```python
from build123d import *

# Parameters (mm, degrees)
F1_DEPTH = 60
F3_DEPTH = 25
F4_R     = 10
F5_DEPTH = 50.8
F7_DEPTH = 42.5
F8_R     = 20


with BuildPart() as f1:
    # F0 (on Front) → F1 (new body)
    with BuildSketch(Plane.XZ):
        with BuildLine():
            Line((94.505748464, -21.1170856844), (94.505748464, -11.1170856844))
            Line((94.505748464, -11.1170856844), (-19.3909259748, -11.1170856844))
            ThreePointArc((-19.3909259748, -11.1170856844), (-22.0195815354, -10.3703397262), (-23.8630619298, -8.3531536619))
            Line((-23.8630619298, -8.3531536619), (-60.860814682, 65.6423518426))
            Line((-60.860814682, 65.6423518426), (-69.805086592, 61.1702158876))
            Line((-69.805086592, 61.1702158876), (-42.972270862, 7.5045844276))
            Line((-42.972270862, 7.5045844276), (-55.494251536, 1.2435940906))
            Line((-55.494251536, 1.2435940906), (-82.327067266, 54.9092255506))
            Line((-82.327067266, 54.9092255506), (-91.271339176, 50.4370895956))
            Line((-91.271339176, 50.4370895956), (-55.494251536, -21.1170856844))
            Line((-55.494251536, -21.1170856844), (94.505748464, -21.1170856844))
        make_face()
    extrude(amount=F1_DEPTH)

    # F2 (on face) → F3 (cut)
    with BuildSketch(Plane.XY.offset(-11.1170856844)):
        with BuildLine():
            Line((94.505748464, -25), (29.505748464, -25))
            ThreePointArc((29.505748464, -25), (24.505748464, -30), (29.505748464, -35))
            Line((29.505748464, -35), (94.505748464, -35))
            Line((94.505748464, -35), (94.505748464, -25))
        make_face()
    extrude(amount=-F3_DEPTH, mode=Mode.SUBTRACT)

    # F4 (on face) → F5 (cut)
    with BuildSketch(Plane(origin=(-22.4317110086, 0, -11.2158555043), x_dir=(0, 1, 0), z_dir=(0.894427191, 0, 0.4472135955))):
        with Locations((-30, 51.9005979594)):
            Circle(F4_R)
    extrude(amount=-F5_DEPTH, mode=Mode.SUBTRACT)

    # F6 (on face) → F7 (cut)
    with BuildSketch(Plane(origin=(-22.4317110086, 0, -11.2158555043), x_dir=(0, 1, 0), z_dir=(0.894427191, 0, 0.4472135955))):
        with BuildLine():
            ThreePointArc((-23.0317006599, 85.9300881282), (-8.8437530091, 78.6280740539), (0, 65.346308328))
            Line((0, 65.346308328), (0, 85.9300881282))
            Line((0, 85.9300881282), (-23.0317006599, 85.9300881282))
        make_face()
        with BuildLine():
            ThreePointArc((-60, 65.346308328), (-51.1562469909, 78.6280740539), (-36.9682993401, 85.9300881282))
            Line((-36.9682993401, 85.9300881282), (-60, 85.9300881282))
            Line((-60, 85.9300881282), (-60, 65.346308328))
        make_face()
    extrude(amount=-F7_DEPTH, mode=Mode.SUBTRACT)

    # F8
    f8_edges = [f1.edges().sort_by_distance(p)[0] for p in [
        (94.505748, 0, -16.117086),
        (94.505748, -60, -16.117086),
    ]]
    fillet(f8_edges, radius=F8_R)


solid = f1.part
```
Design review of the part built by this model. Coordinates are the model's own, in mm. A direction names the side the tool comes from. Give positions to 0.01 mm unless a question says otherwise; leave off trailing zeros. Write each loop counter-clockwise with the first axis right and the second up, starting at its lowest first coordinate (ties: lowest second). Pieces come first, ordered by that corner, then holes. Notation, with made-up numbers: (-3, 66.5) - (7, 66.5) arc R21 ccw to (7, 79.5) - close; hole circle Ø7 at (-12.5, 6.5). An arc over 180 degrees is marked (long way). Return JSON: item names as keys, results as strings. Group by question number.
(1) We need section B-B, the plane y = -27.5. Give the boundary of the cut face in (x, z).
(2) Insertion check: pin 1 (2 mm diameter, centred on x = -24, y = -26.5, fed in from +Z); pin 2 (10 mm diameter, centred on x = 38, y = -26, fed in from +Z); pin 3 (4 mm diameter, centred on x = -65.5, z = 56.5, fed in from +Y); pin 4 (4 mm diameter, centred on x = -34.5, z = -11, fed in from +Y). Each pin has a flat end and moves straight along its axis. Give the tip position at first contact, or say it passes through.
(3) We need section A-A, the plane x = 65. Give the boundary of the cut face in (y, z), then the cut area to 3 significant figures.
(4) Mouldability with a two-part tool opening along X and no side actions: class faces 1 (the cylindrical face through (-21.99, -29.58, -10.39)), 2 (the flat face through (-71.704, -29.58, 33.664)), 3 (the flat face through (-65.27, -29.902, 63.438)) as +X half, -X half, draft (parallel to the pull), parting line (faces both ways), or undercut.
(5) Machinability: for faces 4 (the flat face through (-59.56, -29.58, 40.68)), 5 (the cylindrical face through (88.8, -6.01, -16.05)), 6 (the flat face through (62, -25, -16)), which of the approach directions +Z, -Z, +X, -X, +Y, -Y give a long, thin tool a straight path to every point of the face, cutting with its end or side? Answer none if there is none.
(6) We need section D-D, the plane y = -51. Give the boundary of the cut face in (x, z), then the cut area to 3 significant figures.
(7) We need section C-C, the plane z = 3. Give the boundary of the cut face in (x, y).
(8) To check wall thickness, follow probe 1 along Z at (x, y) = (39, -22.5); probe 2 along X at (y, z) = (-22.5, 54); probe 3 along X at (y, z) = (-42.5, 32). State the ranges of each line that lie inside material, in increasing order.
Reported:
{
 "1": {"outline": "(-91.27, 50.44) - (-80.38, 28.66) - (-71.44, 33.13) - (-82.33, 54.91) - close; (-71.72, 11.34) - (-55.49, -21.12) - (25.18, -21.12) - (25.18, -11.12) - (-19.39, -11.12) arc R5 cw to (-23.86, -8.35) - (-41.31, 26.55) - (-50.26, 22.07) - (-42.97, 7.5) - (-55.49, 1.24) - (-62.78, 15.81) - close; (-69.81, 61.17) - (-58.92, 39.39) - (-49.97, 43.87) - (-60.86, 65.64) - close"},
 "2": {"pin 1": "stops at z = -6.08", "pin 2": "stops at z = -11.12", "pin 3": "stops at y = -7.98", "pin 4": "stops at y = 0"},
 "3": {"outline": "(-60, -21.12) - (-35, -21.12) - (-35, -11.12) - (-60, -11.12) - close; (-25, -21.12) - (0, -21.12) - (0, -11.12) - (-25, -11.12) - close", "area": "500 mm2"},
 "4": {"face 1": "+X half", "face 2": "undercut", "face 3": "-X half"},
 "5": {"face 4": "+Y, -Y", "face 5": "+Z, -Z, +X, +Y", "face 6": "+Z, -Z, +X"},
 "6": {"outline": "(-88.07, 44.03) - (-55.49, -21.12) - (91.21, -21.12) - (91.21, -11.12) - (-19.39, -11.12) arc R5 cw to (-23.86, -8.35) - (-57.66, 59.24) - (-66.6, 54.76) - (-42.97, 7.5) - (-55.49, 1.24) - (-79.12, 48.5) - close", "area": "3,140 mm2"},
 "7": {"outline": "(-67.55, -60) - (-56.37, -60) - (-56.37, 0) - (-67.55, 0) - close; (-51.98, -60) - (-29.54, -60) - (-29.54, 0) - (-51.98, 0) - close"},
 "8": {"probe 1": "z = -21.12 to -11.12", "probe 2": "x = -83.87 to -81.87, -66.22 to -55.04", "probe 3": "x = -82.05 to -70.87, -55.22 to -44.04"}
}
